Here's how the part is built. I have some questions about the finished solid (model axes, mm). A direction names the side the tool comes from. Coordinates: 2 decimals unless noted, no trailing zeros. Order: outer loops, then holes, each group sorted by start corner. A loop starts at its lowest first (then second) coordinate and runs counter-clockwise, first axis right, second up. Notation, with made-up numbers: M 45,59.25 L 56,59.25 A26 cw 56,91.25 Z; hole C 65.25,-0.75 d11. An arc over 180 degrees is marked long. One line per question, with ' | ' between items. Start each with the question number.
```python
from build123d import *

# Parameters (mm, degrees)
SKETCH112_W          = 70.9
SKETCH112_H          = 92.5
PAD067_DEPTH         = 22.2
THICKNESS047_T       = 1.6
SKETCH110_W          = 67.5
SKETCH110_H          = 92.5
PAD066_DEPTH         = 22.2
THICKNESS046_T       = 1.6
SKETCH111_R          = 10
POCKET039_DEPTH      = 22.201
POCKET039_DEPTH_BACK = 1.601
FILLET014_R          = 4
SKETCH108_W          = 67.5
SKETCH108_H          = 92.5
PAD065_DEPTH         = 22.2
THICKNESS045_T       = 1.6
SKETCH109_R          = 10
POCKET038_DEPTH      = 22.201
POCKET038_DEPTH_BACK = 1.601
FILLET015_R          = 4


with BuildPart() as piecestray001:
    # Sketch112 → Pad067 (new body)
    with BuildSketch(Plane.XY):
        Rectangle(SKETCH112_W, SKETCH112_H)
    extrude(amount=PAD067_DEPTH)

    # Thickness047
    thickness047_openings = [piecestray001.faces().sort_by_distance(p)[0] for p in [
        (0, 0, 22.2),
    ]]
    offset(amount=THICKNESS047_T, openings=thickness047_openings, kind=Kind.INTERSECTION)


with BuildPart() as piecestray001_1:
    # Body059 placement: moved
    add(piecestray001.part.moved(Location((70.8, 0, 0))))


with BuildPart() as obj1:
    # Sketch110 → Pad066 (new body)
    with BuildSketch(Plane.XY):
        Rectangle(SKETCH110_W, SKETCH110_H)
    extrude(amount=PAD066_DEPTH)

    # Thickness046
    thickness046_openings = [obj1.faces().sort_by_distance(p)[0] for p in [
        (0, 0, 22.2),
    ]]
    offset(amount=THICKNESS046_T, openings=thickness046_openings, kind=Kind.INTERSECTION)

    # Sketch111 → Pocket039 (cut, two sides)
    with BuildSketch(Plane.XY) as pocket039_sk:
        with Locations((0, -47.85)):
            Circle(SKETCH111_R)
        with Locations((0, 47.85)):
            Circle(SKETCH111_R)
    extrude(amount=POCKET039_DEPTH, mode=Mode.SUBTRACT)
    extrude(pocket039_sk.sketch, amount=-POCKET039_DEPTH_BACK, mode=Mode.SUBTRACT)

    # Fillet014
    fillet014_edges = [obj1.edges().sort_by_distance(p)[0] for p in [
        (9.967741, 47.047411, 22.2),
        (-9.967741, 47.047411, 22.2),
        (-9.967741, -47.047411, 22.2),
        (9.967741, -47.047411, 22.2),
    ]]
    fillet(fillet014_edges, radius=FILLET014_R)


with BuildPart() as obj1_1:
    # Body058 placement: moved
    add(obj1.part.moved(Location((141.6, 0, 0))))


with BuildPart() as obj2:
    # Sketch108 → Pad065 (new body)
    with BuildSketch(Plane.XY):
        Rectangle(SKETCH108_W, SKETCH108_H)
    extrude(amount=PAD065_DEPTH)

    # Thickness045
    thickness045_openings = [obj2.faces().sort_by_distance(p)[0] for p in [
        (0, 0, 22.2),
    ]]
    offset(amount=THICKNESS045_T, openings=thickness045_openings, kind=Kind.INTERSECTION)

    # Sketch109 → Pocket038 (cut, two sides)
    with BuildSketch(Plane.XY) as pocket038_sk:
        with Locations((0, -47.85)):
            Circle(SKETCH109_R)
        with Locations((0, 47.85)):
            Circle(SKETCH109_R)
    extrude(amount=POCKET038_DEPTH, mode=Mode.SUBTRACT)
    extrude(pocket038_sk.sketch, amount=-POCKET038_DEPTH_BACK, mode=Mode.SUBTRACT)

    # Fillet015
    fillet015_edges = [obj2.edges().sort_by_distance(p)[0] for p in [
        (-9.967741, 47.047411, 22.2),
        (-9.967741, -47.047411, 22.2),
        (9.967741, 47.047411, 22.2),
        (9.967741, -47.047411, 22.2),
    ]]
    fillet(fillet015_edges, radius=FILLET015_R)

    # Boolean002: union PiecesTray001, obj1
    add(piecestray001_1.part)
    add(obj1_1.part)


solid = obj2.part
```
1. Imagine slicing it at A-A (z = 7). Count the separate pieces of the cut face and the enclosed holes in it, then the cut area to 3 significant figures.
2. Imagine slicing it at C-C (x = 75.5). List the corners of the cut face in (y, z) for me.
3. We'd pull the mould along Y, two halves only. Please class faces 3 (the face through (107.85, -1, 11)), 4 (the face through (-34, 14, 22.2)), 5 (the face through (164, -47.85, 10)): released by +Y, released by -Y, zero draft, split by the parting line, or undercut.
4. Imagine slicing it at B-B (y = -42). List the corners of the cut face in (x, z) for me, then the cut area to 3 significant figures.
5. Imagine slicing it at D-D (y = 22.5). List the corners of the cut face in (x, z) for me.
6. Will this pin go through, and if not, where does the flat tip stop? pin 1 (1 mm diameter, centred on x = 148, y = 3.5, fed in from +Z).
7. Which directions (+Z, -Z, +X, -X, +Y, -Y) give clear straight access to the entire face, cutting with the end or side of a thin tool? Please do faces 1 (the face through (70, 46.25, 11)), 2 (the face through (164, 47.85, 10)).
8. I need wall thicknesses on line 1 (X direction, y = 6.5, z = 1); line 2 (Y direction, x = 72, z = 19). Which ranges of each line are inside material? Lowest first, please.
Entries:
1) separate pieces: 3 | enclosed holes: 1 | area: 1,140 mm²
2) outline: M -47.85,-1.6 L 47.85,-1.6 L 47.85,22.2 L 46.25,22.2 L 46.25,0 L -46.25,0 L -46.25,22.2 L -47.85,22.2 Z
3) face 3: undercut | face 4: zero draft | face 5: released by -Y
4) outline: M -35.35,-1.6 L -8.11,-1.6 L -8.11,0 L -33.75,0 L -33.75,22.2 L -35.35,22.2 Z; M 8.11,-1.6 L 133.49,-1.6 L 133.49,0 L 107.85,0 L 107.85,22.2 L 106.25,22.2 L 106.25,0 L 35.35,0 L 35.35,22.2 L 33.75,22.2 L 33.75,0 L 8.11,0 Z; M 149.71,-1.6 L 176.95,-1.6 L 176.95,22.2 L 175.35,22.2 L 175.35,0 L 149.71,0 Z | area: 430 mm²
5) outline: M -35.35,-1.6 L 176.95,-1.6 L 176.95,22.2 L 175.35,22.2 L 175.35,0 L 107.85,0 L 107.85,22.2 L 106.25,22.2 L 106.25,0 L 35.35,0 L 35.35,22.2 L 33.75,22.2 L 33.75,0 L -33.75,0 L -33.75,22.2 L -35.35,22.2 Z
6) pin 1: z = 0
7) face 1: +Z | face 2: +Z, -Z, +X, -X, +Y
8) line 1: -35.35 to -33.75, 33.75 to 35.35, 106.25 to 107.85, 175.35 to 176.95 | line 2: -47.85 to -46.25, 46.25 to 47.85
